from build123d import *

# Parameters (mm, degrees)
SKETCH1_W                                   = 76.2
SKETCH1_H                                   = 76.2
BOSS_EXTRUDE1_DEPTH                         = 127
FILLET1_R                                   = 12.7
SKETCH2_W                                   = 76.2
SKETCH2_H                                   = 12.7
BOSS_EXTRUDE6_DEPTH                         = 57.15
CUT_EXTRUDE2_DEPTH                          = 12.7
CUT_EXTRUDE4_START                          = -254
SKETCH6_W                                   = 71.12
SKETCH6_H                                   = 16.51
SKETCH6_H_2                                 = 17.78
SKETCH6_R                                   = 6.35
CUT_EXTRUDE4_DEPTH                          = 254
SKETCH7_W                                   = 50.8
SKETCH7_H                                   = 10.16
CUT_EXTRUDE7_DEPTH                          = 124.46
CUT_EXTRUDE8_DEPTH                          = 114.3
BOSS_EXTRUDE7_DEPTH                         = 12.7
SKETCH7_8_W                                 = 50.8
SKETCH7_8_H                                 = 10.16
CUT_EXTRUDE9_DEPTH                          = 127
CBORE_FOR_1_BINDING_HEAD_MACHINE_SC_2_COUNT = 2
CBORE_FOR_1_BINDING_HEAD_MACHINE_SC_2_PITCH = 38.1
CBORE_FOR_1_BINDING_HEAD_MACHINE_SC_3_COUNT = 2
CBORE_FOR_1_BINDING_HEAD_MACHINE_SC_3_PITCH = 114.3
CBORE_FOR_1_BINDING_HEAD_MACHINE_SC_4_COUNT = 2
CBORE_FOR_1_BINDING_HEAD_MACHINE_SC_4_PITCH = 120.482778852


with BuildPart() as part:
    # Sketch1 → Boss-Extrude1 (new body)
    with BuildSketch(Plane(origin=(0, 0, 0), x_dir=(1, 0, 0), z_dir=(0, 1, 0))):
        Rectangle(SKETCH1_W, SKETCH1_H)
    extrude(amount=BOSS_EXTRUDE1_DEPTH)

    # Fillet1
    fillet1_edges = [part.edges().sort_by_distance(p)[0] for p in [
        (38.1, 63.5, 38.1),
        (-38.1, 63.5, 38.1),
        (-38.1, 63.5, -38.1),
        (38.1, 63.5, -38.1),
    ]]
    fillet(fillet1_edges, radius=FILLET1_R)

    # Sketch2 → Boss-Extrude6 (add)
    with BuildSketch(Plane(origin=(0, 127, 0), x_dir=(1, 0, 0), z_dir=(0, 1, 0))):
        Rectangle(SKETCH2_W, SKETCH2_H)
    extrude(amount=BOSS_EXTRUDE6_DEPTH)

    # Sketch5 → Cut-Extrude2 (cut)
    with BuildSketch(Plane.XY.offset(6.35)):
        with BuildLine():
            Line((-38.1, 184.15), (-38.1, 146.05))
            ThreePointArc((-38.1, 146.05), (-26.940768363, 172.990768363), (0, 184.15))
            Line((0, 184.15), (-38.1, 184.15))
        make_face()
        with BuildLine():
            ThreePointArc((0, 173.99), (-17.329273527, 167.96665757), (-27.186811297, 152.493670653))
            Line((-27.186811297, 152.493670653), (0, 152.493670653))
            Line((0, 152.493670653), (0, 173.99))
        make_face()
        with BuildLine():
            Line((0, 173.99), (0, 152.493670653))
            Line((0, 152.493670653), (27.186811297, 152.493670653))
            ThreePointArc((27.186811297, 152.493670653), (17.329273527, 167.96665757), (0, 173.99))
        make_face()
        with BuildLine():
            Line((-27.94, 146.05), (-27.94, 132.743180509))
            ThreePointArc((-27.94, 132.743180509), (-21.337126939, 140.622484939), (-12.60652265, 146.05))
            Line((-12.60652265, 146.05), (-27.94, 146.05))
        make_face()
        with BuildLine():
            ThreePointArc((12.60652265, 146.05), (21.337126939, 140.622484939), (27.94, 132.743180509))
            Line((27.94, 132.743180509), (27.94, 146.05))
            Line((27.94, 146.05), (12.60652265, 146.05))
        make_face()
        with BuildLine():
            ThreePointArc((0, 146.05), (-16.908179234, 140.834329543), (-27.94, 127))
            Line((-27.94, 127), (27.94, 127))
            ThreePointArc((27.94, 127), (16.908179234, 140.834329543), (0, 146.05))
        make_face()
        with BuildLine():
            ThreePointArc((0, 184.15), (26.940768363, 172.990768363), (38.1, 146.05))
            Line((38.1, 146.05), (38.1, 184.15))
            Line((38.1, 184.15), (0, 184.15))
        make_face()
    extrude(amount=-CUT_EXTRUDE2_DEPTH, mode=Mode.SUBTRACT)

    # Sketch6 → Cut-Extrude4 (cut)
    # profile 1 of 5: a face of its own
    with BuildSketch(Plane.XZ.offset(CUT_EXTRUDE4_START)):
        with Locations((0, 17.145)):
            Rectangle(SKETCH6_W, SKETCH6_H)
    # profile 2 of 5: a face of its own
    with BuildSketch(Plane.XZ.offset(CUT_EXTRUDE4_START)):
        with BuildLine():
            Line((-35.56, 25.4), (-38.1, 25.4))
            Line((-38.1, 25.4), (-38.1, -25.4))
            ThreePointArc((-38.1, -25.4), (-34.380256121, -34.380256121), (-25.4, -38.1))
            Line((-25.4, -38.1), (25.4, -38.1))
            ThreePointArc((25.4, -38.1), (34.380256121, -34.380256121), (38.1, -25.4))
            Line((38.1, -25.4), (38.1, 25.4))
            Line((38.1, 25.4), (35.56, 25.4))
            Line((35.56, 25.4), (35.56, 8.89))
            Line((35.56, 8.89), (35.56, -8.89))
            Line((35.56, -8.89), (35.56, -25.4))
            ThreePointArc((35.56, -25.4), (32.584204897, -32.584204897), (25.4, -35.56))
            Line((25.4, -35.56), (-25.4, -35.56))
            ThreePointArc((-25.4, -35.56), (-32.584204897, -32.584204897), (-35.56, -25.4))
            Line((-35.56, -25.4), (-35.56, -8.89))
            Line((-35.56, -8.89), (-35.56, 8.89))
            Line((-35.56, 8.89), (-35.56, 25.4))
        make_face()
    # profile 3 of 5: a face of its own
    with BuildSketch(Plane.XZ.offset(CUT_EXTRUDE4_START)):
        Rectangle(SKETCH6_W, SKETCH6_H_2)
        Circle(SKETCH6_R, mode=Mode.SUBTRACT)
    # profile 4 of 5: a face of its own
    with BuildSketch(Plane.XZ.offset(CUT_EXTRUDE4_START)):
        Circle(SKETCH6_R)
    # profile 5 of 5: a face of its own
    with BuildSketch(Plane.XZ.offset(CUT_EXTRUDE4_START)):
        with BuildLine():
            Line((35.56, -8.89), (-35.56, -8.89))
            Line((-35.56, -8.89), (-35.56, -25.4))
            ThreePointArc((-35.56, -25.4), (-32.584204897, -32.584204897), (-25.4, -35.56))
            Line((-25.4, -35.56), (25.4, -35.56))
            ThreePointArc((25.4, -35.56), (32.584204897, -32.584204897), (35.56, -25.4))
            Line((35.56, -25.4), (35.56, -8.89))
        make_face()
    extrude(amount=CUT_EXTRUDE4_DEPTH, mode=Mode.SUBTRACT)

    # Sketch7 → Cut-Extrude7 (cut)
    with BuildSketch(Plane.XZ):
        with Locations((0, 30.48)):
            Rectangle(SKETCH7_W, SKETCH7_H)
    extrude(amount=-CUT_EXTRUDE7_DEPTH, mode=Mode.SUBTRACT)

    # Sketch7_6 → Cut-Extrude8 (cut)
    with BuildSketch(Plane.XZ):
        with BuildLine():
            ThreePointArc((-25.4, 35.56), (-32.584204897, 32.584204897), (-35.56, 25.4))
            Line((-35.56, 25.4), (-25.4, 25.4))
            Line((-25.4, 25.4), (-25.4, 35.56))
        make_face()
        with BuildLine():
            Line((25.4, 35.56), (25.4, 25.4))
            Line((25.4, 25.4), (35.56, 25.4))
            ThreePointArc((35.56, 25.4), (32.584204897, 32.584204897), (25.4, 35.56))
        make_face()
    extrude(amount=-CUT_EXTRUDE8_DEPTH, mode=Mode.SUBTRACT)

    # Sketch7_7 → Boss-Extrude7 (add)
    with BuildSketch(Plane.XZ):
        with BuildLine():
            ThreePointArc((-25.4, 35.56), (-32.584204897, 32.584204897), (-35.56, 25.4))
            Line((-35.56, 25.4), (-25.4, 25.4))
            Line((-25.4, 25.4), (-25.4, 35.56))
        make_face()
        with BuildLine():
            Line((25.4, 35.56), (25.4, 25.4))
            Line((25.4, 25.4), (35.56, 25.4))
            ThreePointArc((35.56, 25.4), (32.584204897, 32.584204897), (25.4, 35.56))
        make_face()
    extrude(amount=-BOSS_EXTRUDE7_DEPTH)

    # Sketch7_8 → Cut-Extrude9 (cut)
    with BuildSketch(Plane.XZ):
        with BuildLine():
            Line((25.4, 35.56), (25.4, 25.4))
            Line((25.4, 25.4), (35.56, 25.4))
            ThreePointArc((35.56, 25.4), (32.584204897, 32.584204897), (25.4, 35.56))
        make_face()
        with Locations((0, 30.48)):
            Rectangle(SKETCH7_8_W, SKETCH7_8_H)
        with BuildLine():
            ThreePointArc((-25.4, 35.56), (-32.584204897, 32.584204897), (-35.56, 25.4))
            Line((-35.56, 25.4), (-25.4, 25.4))
            Line((-25.4, 25.4), (-25.4, 35.56))
        make_face()
    extrude(amount=-CUT_EXTRUDE9_DEPTH, mode=Mode.SUBTRACT)

    # Sketch12 → CBORE for _1 Binding Head Machine Screw1 (revolve, cut)
    with BuildSketch(Plane(origin=(-19.05, 120.65, 38.1), x_dir=(0, -1, 0), z_dir=(1, 0, 0))):
        Polygon((0, 0), (0, 10.839152758), (1.1303, 10.16), (1.1303, 1.0414), (2.38125, 1.0414), (2.38125, 0.532828266), (3.01625, 0), align=None)
    cbore_for_1_binding_head_machine_screw1 = revolve(axis=Axis((-19.05, 120.65, 44.45), (0, 0, -1)), mode=Mode.SUBTRACT)

    # CBORE for _1 Binding Head Machine Sc 2: CBORE for _1 Binding Head Machine Screw1 ×2
    with Locations(*[(i * CBORE_FOR_1_BINDING_HEAD_MACHINE_SC_2_PITCH, 0, 0) for i in range(1, CBORE_FOR_1_BINDING_HEAD_MACHINE_SC_2_COUNT)]):
        add(cbore_for_1_binding_head_machine_screw1, mode=Mode.SUBTRACT)

    # CBORE for _1 Binding Head Machine Sc 3: CBORE for _1 Binding Head Machine Screw1 ×2
    with Locations(*[(0, -i * CBORE_FOR_1_BINDING_HEAD_MACHINE_SC_3_PITCH, 0) for i in range(1, CBORE_FOR_1_BINDING_HEAD_MACHINE_SC_3_COUNT)]):
        add(cbore_for_1_binding_head_machine_screw1, mode=Mode.SUBTRACT)

    # CBORE for _1 Binding Head Machine Sc 4: CBORE for _1 Binding Head Machine Screw1 ×2
    with Locations(*[Vector(0.3162277660168378, -0.9486832980505139, 0) * (i * CBORE_FOR_1_BINDING_HEAD_MACHINE_SC_4_PITCH) for i in range(1, CBORE_FOR_1_BINDING_HEAD_MACHINE_SC_4_COUNT)]):
        add(cbore_for_1_binding_head_machine_screw1, mode=Mode.SUBTRACT)


solid = part.part
Check sheet for the modelled part. Datum: model origin and axes. Units: mm. A direction names the side the tool comes from. Round coordinates to 2 decimals unless told otherwise and drop trailing zeros. Order: outer loops, then holes, each group sorted by start corner. A loop starts at its lowest first (then second) coordinate and runs counter-clockwise, first axis right, second up.
(1) Cross-section at A-A, the plane y = 51. Enter the section's corners in (x, z).
(2) Go/stop test with flat-tipped pins: P1, Ø5.5, axis at x = 19.05, y = 6.35, coming from the +Z side; P2, Ø4.5, axis at x = -19.05, y = 120.65, coming from the +Z side; P3, Ø2, axis at y = 35, z = 32, coming from the +X side; P4, Ø1.5, axis at x = 28.5, z = 33.5, coming from the -Y side. Record where each tip stops, or that it passes through.
(3) Scan lines: probe 1 along Y at (x, z) = (19.05, 37.45); probe 2 along Y at (x, z) = (-19.05, 36.1); probe 3 along X at (y, z) = (6.35, 36.6). Record each from-to range of solid material in increasing order.
(4) Cross-section at D-D, the plane x = 30.5. Enter the section's corners in (y, z).
(5) Access from +Z, -Z, +X, -X, +Y, -Y to the whole of each face (thin tool, end or side, straight path). Record for faces 3 (the cylindrical face through (32.663, 62.611, 32.505)), 4 (the cylindrical face through (-16.94, 5.25, 37.32)), 5 (the cylindrical face through (34.28, 64.39, 34.48)).
(6) Cross-section at C-C, the plane x = 3. Enter the section's corners in (y, z).
(7) Cross-section at B-B, the plane z = 30. Enter the section's corners in (x, y), and give its area (3 significant figures).
(8) Draft check along Y on faces 1 (the cylindrical face through (-19.814, 7.183, 36.32)), 2 (the flat face through (-37, 63, 25.4)). Enter one of: pulls with the +Y half, pulls with the -Y half, needs draft (parallel to the pull), parting line crosses it, or undercut.
Check sheet entries:
1. outline: (-38.1, 25.4) - (-35.56, 25.4) arc R10.16 cw to (-25.4, 35.56) - (25.4, 35.56) arc R10.16 cw to (35.56, 25.4) - (38.1, 25.4) arc R12.7 ccw to (25.4, 38.1) - (-25.4, 38.1) arc R12.7 ccw to start
2. P1: stops at z = 37.88
2. P2: stops at z = 37.06
2. P3: stops at x = 36.8
2. P4: passes through
3. probe 1: y = 0 to 3.97, 8.73 to 118.27, 123.03 to 127
3. probe 2: y = 0 to 5.22, 7.48 to 119.52, 121.78 to 127
3. probe 3: x = -31.39 to -20.18, -17.92 to 17.92, 20.18 to 31.39
4. outline: (0, 34.19) - (127, 34.19) - (127, 37.03) - (0, 37.03) - close
5. face 3: -Z, +Y, -Y
5. face 4: +Z
5. face 5: +Z, +X, +Y, -Y
6. outline: (0, 35.56) - (127, 35.56) - (127, 38.1) - (0, 38.1) - close
7. outline: (-37.24, 0) - (-34.46, 0) - (-34.46, 127) - (-37.24, 127) - close; (34.46, 0) - (37.24, 0) - (37.24, 127) - (34.46, 127) - close
7. area: 706 mm2
8. face 1: undercut
8. face 2: needs draft
